```python
from build123d import *

# Parameters (mm, degrees)
ESQUISSE1_W             = 100
ESQUISSE1_H             = 200
BOSS_EXTRU_1_DEPTH      = 6
ESQUISSE2_R             = 2
ESQUISSE2_R_2           = 4
ENL_V_MAT_EXTRU_1_DEPTH = 6
CONG_1_R                = 20


with BuildPart() as part:
    # Esquisse1 → Boss.-Extru.1 (new body)
    with BuildSketch(Plane.XY):
        with Locations((-130.633802817, 58.529929577)):
            Rectangle(ESQUISSE1_W, ESQUISSE1_H)
    extrude(amount=BOSS_EXTRU_1_DEPTH)

    # Esquisse2 → Enlèv. mat.-Extru.1 (cut)
    with BuildSketch(Plane.XY.offset(6)):
        with Locations((-166.633802817, 94.529929577)):
            Circle(ESQUISSE2_R)
        with Locations((-166.633802817, 22.529929577)):
            Circle(ESQUISSE2_R)
        with Locations((-94.633802817, 22.529929577)):
            Circle(ESQUISSE2_R)
        with Locations((-94.633802817, 94.529929577)):
            Circle(ESQUISSE2_R)
        with Locations((-130.633802817, 138.529929577)):
            Circle(ESQUISSE2_R_2)
        with Locations((-130.633802817, -21.470070423)):
            Circle(ESQUISSE2_R_2)
    extrude(amount=-ENL_V_MAT_EXTRU_1_DEPTH, mode=Mode.SUBTRACT)

    # Congé1
    cong_1_edges = [part.edges().sort_by_distance(p)[0] for p in [
        (-180.633802817, 158.529929577, 3),
        (-80.633802817, 158.529929577, 3),
        (-80.633802817, -41.470070423, 3),
        (-180.633802817, -41.470070423, 3),
    ]]
    fillet(cong_1_edges, radius=CONG_1_R)


solid = part.part
```
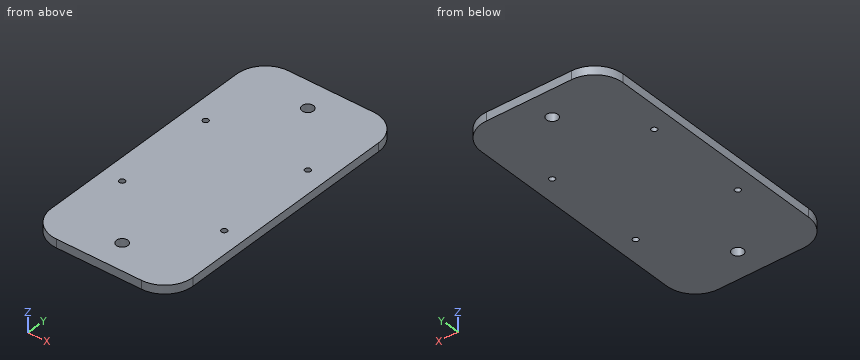
Geometry: final body of the model. Coordinates: model frame, mm. Round coordinates to 2 decimals unless told otherwise and drop trailing zeros. Loops run counter-clockwise (first coordinate to the right, second up) from the corner with the lowest first, then second, coordinate; pieces in that order, holes last. Notation, with made-up numbers: (18, -15) -> (73, -15) arc R22 cw to (73, 23) -> close; hole circle Ø2 at (18, 61.5). An arc over 180 degrees is marked (long way). Use one line per item in the form item = value.
Item 1: Cut plane C-C on x = -166.5. Output: boundary loops of the cut face in (y, z).
Evaluation:
outline = (-40.59, 0) -> (20.53, 0) -> (20.53, 6) -> (-40.59, 6) -> close; (24.53, 0) -> (92.53, 0) -> (92.53, 6) -> (24.53, 6) -> close; (96.53, 0) -> (157.65, 0) -> (157.65, 6) -> (96.53, 6) -> close
Item 2: Contact query for flat-ended pins moving along their axis: pin 1 Ø2 at (x, z) = (-95, 3.5) entering from +Y; pin 2 Ø1.5 at (x, z) = (-96.5, 4.5) entering from -Y. Output: stop coordinate, or through.
Evaluation:
pin_1 = 157.99
pin_2 = -41.18
Item 3: Cut plane A-A on x = -132. Output: boundary loops of the cut face in (y, z), then the cut area to 3 significant figures.
Evaluation:
outline = (-41.47, 0) -> (-25.23, 0) -> (-25.23, 6) -> (-41.47, 6) -> close; (-17.71, 0) -> (134.77, 0) -> (134.77, 6) -> (-17.71, 6) -> close; (142.29, 0) -> (158.53, 0) -> (158.53, 6) -> (142.29, 6) -> close
area = 1,110 mm2
Item 4: Material intervals for probe 1 along X at (y, z) = (135, 4.9); probe 2 along X at (y, z) = (146, 4.4); probe 3 along Y at (x, z) = (-175, 3.9), sorted ascending.
Evaluation:
probe_1 = -180.63 to -132.52, -128.75 to -80.63
probe_2 = -179.19 to -82.08
probe_3 = -35.38 to 152.44
Item 5: Cut plane B-B on z = 3.2. Output: boundary loops of the cut face in (x, y).
Evaluation:
outline = (-180.63, -21.47) arc R20 ccw to (-160.63, -41.47) -> (-100.63, -41.47) arc R20 ccw to (-80.63, -21.47) -> (-80.63, 138.53) arc R20 ccw to (-100.63, 158.53) -> (-160.63, 158.53) arc R20 ccw to (-180.63, 138.53) -> close; hole circle Ø4 at (-166.63, 22.53); hole circle Ø4 at (-166.63, 94.53); hole circle Ø8 at (-130.63, -21.47); hole circle Ø8 at (-130.63, 138.53); hole circle Ø4 at (-94.63, 22.53); hole circle Ø4 at (-94.63, 94.53)
